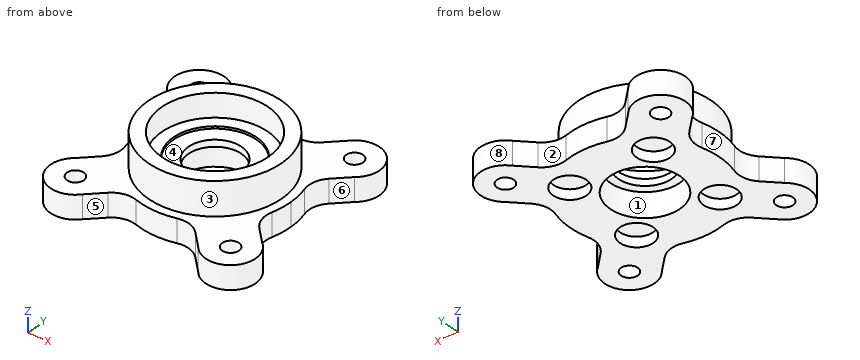
```python
from build123d import *

# Parameters (mm, degrees)
SKETCH1_R                             = 7.5
SKETCH1_R_2                           = 22.5
F_5_IN_SHEET_DEPTH                    = 7
FILLET1_R                             = 7
F_5_0_REAMED_OVER_FOR_SHOULDER_BOLT_D = 5
SKETCH8_R                             = 20
BOSS_EXTRUDE2_DEPTH                   = 10
SKETCH2_R                             = 8
THROUGH_HOLE_DEPTH                    = 47.337664072
SKETCH7_R                             = 10.5
INBOARD_BEARING_CUP_DEPTH             = 7.325
SKETCH11_R                            = 12.5
CUT_EXTRUDE5_DEPTH                    = 7.675
SKETCH12_R                            = 16
CUT_EXTRUDE6_DEPTH                    = 7
SKETCH13_R                            = 5
CUT_EXTRUDE7_DEPTH                    = 3


with BuildPart() as part:
    # Sketch1 → .5 in sheet (new body)
    with BuildSketch(Plane.XY):
        with Locations((22.980970389, 22.980970389)):
            Circle(SKETCH1_R)
        Circle(SKETCH1_R_2)
        with Locations((-22.980970389, 22.980970389)):
            Circle(SKETCH1_R)
        with Locations((-22.980970389, -22.980970389)):
            Circle(SKETCH1_R)
        with Locations((22.980970389, -22.980970389)):
            Circle(SKETCH1_R)
        with BuildLine():
            ThreePointArc((-17.10117153, 27.636930588), (-28.284271247, 28.284271247), (-27.636930588, 17.10117153))
            Line((-27.636930588, 17.10117153), (-17.10117153, 27.636930588))
        make_face()
        with BuildLine():
            Line((-17.10117153, 27.636930588), (-27.636930588, 17.10117153))
            ThreePointArc((-27.636930588, 17.10117153), (-19.715216379, 16.229314981), (-15.480970389, 22.980970389))
            ThreePointArc((-15.480970389, 22.980970389), (-15.897592259, 25.445874906), (-17.10117153, 27.636930588))
        make_face()
        with BuildLine():
            Line((-27.636930588, 17.10117153), (-20.280355849, 9.744596791))
            ThreePointArc((-20.280355849, 9.744596791), (-15.909902577, 15.909902577), (-9.744596791, 20.280355849))
            Line((-9.744596791, 20.280355849), (-17.10117153, 27.636930588))
            ThreePointArc((-17.10117153, 27.636930588), (-15.897592259, 25.445874906), (-15.480970389, 22.980970389))
            ThreePointArc((-15.480970389, 22.980970389), (-19.715216379, 16.229314981), (-27.636930588, 17.10117153))
        make_face()
        with BuildLine():
            Line((-20.280355849, 9.744596791), (-10.535759058, 0))
            Line((-10.535759058, 0), (0, 10.535759058))
            Line((0, 10.535759058), (-9.744596791, 20.280355849))
            ThreePointArc((-9.744596791, 20.280355849), (-15.909902577, 15.909902577), (-20.280355849, 9.744596791))
        make_face()
        with BuildLine():
            Line((-9.744596791, 20.280355849), (0, 10.535759058))
            Line((0, 10.535759058), (9.744596791, 20.280355849))
            ThreePointArc((9.744596791, 20.280355849), (0, 22.5), (-9.744596791, 20.280355849))
        make_face()
        with BuildLine():
            Line((-20.280355849, -9.744596791), (-10.535759058, 0))
            Line((-10.535759058, 0), (-20.280355849, 9.744596791))
            ThreePointArc((-20.280355849, 9.744596791), (-22.5, 0), (-20.280355849, -9.744596791))
        make_face()
        with BuildLine():
            ThreePointArc((-9.744596791, -20.280355849), (0, -22.5), (9.744596791, -20.280355849))
            Line((9.744596791, -20.280355849), (0, -10.535759058))
            Line((0, -10.535759058), (-9.744596791, -20.280355849))
        make_face()
        with BuildLine():
            Line((0, -10.535759058), (9.744596791, -20.280355849))
            ThreePointArc((9.744596791, -20.280355849), (15.909902577, -15.909902577), (20.280355849, -9.744596791))
            Line((20.280355849, -9.744596791), (10.535759058, 0))
            Line((10.535759058, 0), (0, -10.535759058))
        make_face()
        with BuildLine():
            Line((10.535759058, 0), (20.280355849, -9.744596791))
            ThreePointArc((20.280355849, -9.744596791), (21.938072005, -4.997098828), (22.5, 0))
            ThreePointArc((22.5, 0), (21.938072005, 4.997098828), (20.280355849, 9.744596791))
            Line((20.280355849, 9.744596791), (10.535759058, 0))
        make_face()
        with BuildLine():
            Line((0, 10.535759058), (10.535759058, 0))
            Line((10.535759058, 0), (20.280355849, 9.744596791))
            ThreePointArc((20.280355849, 9.744596791), (15.909902577, 15.909902577), (9.744596791, 20.280355849))
            Line((9.744596791, 20.280355849), (0, 10.535759058))
        make_face()
        Polygon((-10.535759058, 0), (0, -10.535759058), (10.535759058, 0), (0, 10.535759058), align=None)
        with BuildLine():
            ThreePointArc((17.10117153, 27.636930588), (17.67766953, 17.67766953), (27.636930588, 17.10117153))
            Line((27.636930588, 17.10117153), (17.10117153, 27.636930588))
        make_face()
        with BuildLine():
            Line((17.10117153, 27.636930588), (27.636930588, 17.10117153))
            ThreePointArc((27.636930588, 17.10117153), (29.732625796, 19.715216379), (30.480970389, 22.980970389))
            ThreePointArc((30.480970389, 22.980970389), (25.445874906, 30.064348518), (17.10117153, 27.636930588))
        make_face()
        with BuildLine():
            ThreePointArc((9.744596791, 20.280355849), (15.909902577, 15.909902577), (20.280355849, 9.744596791))
            Line((20.280355849, 9.744596791), (27.636930588, 17.10117153))
            ThreePointArc((27.636930588, 17.10117153), (17.67766953, 17.67766953), (17.10117153, 27.636930588))
            Line((17.10117153, 27.636930588), (9.744596791, 20.280355849))
        make_face()
        with BuildLine():
            ThreePointArc((27.636930588, -17.10117153), (17.67766953, -17.67766953), (17.10117153, -27.636930588))
            Line((17.10117153, -27.636930588), (27.636930588, -17.10117153))
        make_face()
        with BuildLine():
            Line((27.636930588, -17.10117153), (17.10117153, -27.636930588))
            ThreePointArc((17.10117153, -27.636930588), (25.445874906, -30.064348518), (30.480970389, -22.980970389))
            ThreePointArc((30.480970389, -22.980970389), (29.732625796, -19.715216379), (27.636930588, -17.10117153))
        make_face()
        with BuildLine():
            Line((9.744596791, -20.280355849), (17.10117153, -27.636930588))
            ThreePointArc((17.10117153, -27.636930588), (17.67766953, -17.67766953), (27.636930588, -17.10117153))
            Line((27.636930588, -17.10117153), (20.280355849, -9.744596791))
            ThreePointArc((20.280355849, -9.744596791), (15.909902577, -15.909902577), (9.744596791, -20.280355849))
        make_face()
        with BuildLine():
            ThreePointArc((-27.636930588, -17.10117153), (-28.284271247, -28.284271247), (-17.10117153, -27.636930588))
            Line((-17.10117153, -27.636930588), (-27.636930588, -17.10117153))
        make_face()
        with BuildLine():
            Line((-27.636930588, -17.10117153), (-17.10117153, -27.636930588))
            ThreePointArc((-17.10117153, -27.636930588), (-15.897592259, -25.445874906), (-15.480970389, -22.980970389))
            ThreePointArc((-15.480970389, -22.980970389), (-19.715216379, -16.229314981), (-27.636930588, -17.10117153))
        make_face()
        with BuildLine():
            Line((-17.10117153, -27.636930588), (-9.744596791, -20.280355849))
            ThreePointArc((-9.744596791, -20.280355849), (-15.909902577, -15.909902577), (-20.280355849, -9.744596791))
            Line((-20.280355849, -9.744596791), (-27.636930588, -17.10117153))
            ThreePointArc((-27.636930588, -17.10117153), (-19.715216379, -16.229314981), (-15.480970389, -22.980970389))
            ThreePointArc((-15.480970389, -22.980970389), (-15.897592259, -25.445874906), (-17.10117153, -27.636930588))
        make_face()
    extrude(amount=F_5_IN_SHEET_DEPTH)

    # Fillet1
    fillet1_edges = [part.edges().sort_by_distance(p)[0] for p in [
        (-9.744596791, -20.280355849, 3.5),
        (-20.280355849, -9.744596791, 3.5),
        (-20.280355849, 9.744596791, 3.5),
        (-9.744596791, 20.280355849, 3.5),
        (9.744596791, 20.280355849, 3.5),
        (20.280355849, 9.744596791, 3.5),
        (20.280355849, -9.744596791, 3.5),
        (9.744596791, -20.280355849, 3.5),
    ]]
    fillet(fillet1_edges, radius=FILLET1_R)

    # Ø5.0 Reamed over for shoulder bolt (through all)
    with Locations(Plane(origin=(-11.055401524, 12.777106872, 7), x_dir=(1, 0, 0), z_dir=(0, 0, 1))):
        with Locations((-11.925568864, 10.203863517), (34.036371913, 10.203863517), (34.036371913, -35.758077261), (-11.925568864, -35.758077261)):
            Hole(F_5_0_REAMED_OVER_FOR_SHOULDER_BOLT_D / 2)

    # Sketch8 → Boss-Extrude2 (add)
    with BuildSketch(Plane.XY.offset(7)):
        Circle(SKETCH8_R)
    extrude(amount=BOSS_EXTRUDE2_DEPTH)

    # Sketch2 → Through hole (cut, through all)
    with BuildSketch(Plane.XY):
        Circle(SKETCH2_R)
    extrude(amount=THROUGH_HOLE_DEPTH, mode=Mode.SUBTRACT)

    # Sketch7 → Inboard bearing cup (cut)
    with BuildSketch(Plane(origin=(0, 0, 0), x_dir=(-1, 0, 0), z_dir=(0, 0, -1))):
        Circle(SKETCH7_R)
    extrude(amount=-INBOARD_BEARING_CUP_DEPTH, mode=Mode.SUBTRACT)

    # Sketch11 → Cut-Extrude5 (cut)
    with BuildSketch(Plane.XY.offset(17)):
        Circle(SKETCH11_R)
    extrude(amount=-CUT_EXTRUDE5_DEPTH, mode=Mode.SUBTRACT)

    # Sketch12 → Cut-Extrude6 (cut)
    with BuildSketch(Plane.XY.offset(17)):
        Circle(SKETCH12_R)
    extrude(amount=-CUT_EXTRUDE6_DEPTH, mode=Mode.SUBTRACT)

    # Sketch13 → Cut-Extrude7 (cut)
    with BuildSketch(Plane(origin=(0, 0, 0), x_dir=(-1, 0, 0), z_dir=(0, 0, -1))):
        with Locations((12.374368671, 12.374368671)):
            Circle(SKETCH13_R)
        with Locations((-12.374368671, 12.374368671)):
            Circle(SKETCH13_R)
        with Locations((-12.374368671, -12.374368671)):
            Circle(SKETCH13_R)
        with Locations((12.374368671, -12.374368671)):
            Circle(SKETCH13_R)
    extrude(amount=-CUT_EXTRUDE7_DEPTH, mode=Mode.SUBTRACT)


solid = part.part
```
Verification items for the finished model (mm, model axes). Face numbers are marked on the shaded views. A direction names the side the tool comes from. Round coordinates to 2 decimals unless told otherwise and drop trailing zeros. Write each loop counter-clockwise with the first axis right and the second up, starting at its lowest first coordinate (ties: lowest second). Pieces come first, ordered by that corner, then holes.
1. Scan lines: L1, parallel to Y at x = 24.5, z = 2; L2, parallel to X at y = 0.5, z = 10.25; L3, parallel to Y at x = 24, z = 1. Record each from-to range of solid material in increasing order.
2. Gauge pin test, flat ends, axial feed: P1, Ø3, axis at x = 11, y = 10.5, coming from the -Z side; P2, Ø8, axis at x = -1.5, y = 6, coming from the +Z side (3 decimals); P3, Ø8, axis at x = -22.98, y = 22.98, coming from the +Z side. Record the tip position at first contact, or that the pin passes through.
3. Draft check along Y on the marked faces 1, 2 and 3. Enter one of: +Y half, -Y half, draft (parallel to the pull), parting line (faces both ways), or undercut.
4. Section check B-B on z = 14.5. Enter the section's corners in (x, y).
5. Section check A-A on x = 0. Enter the section's corners in (y, z) (3 decimals), plus the area to 3 significant figures.
6. Section check C-C on y = -11.5. Enter the section's corners in (x, z) (3 decimals).
7. Section check D-D on x = -14.5. Enter the section's corners in (y, z).
8. Access from +Z, -Z, +X, -X, +Y, -Y to the whole of each face (thin tool, end or side, straight path). Record for the marked faces 4, 5, 6, 7 and 8.
Answer:
1. L1: y = -30.33 to -24.97, -21 to -13.96, 13.96 to 21, 24.97 to 30.33
1. L2: x = -19.99 to -15.99, 15.99 to 19.99
1. L3: y = -30.41 to -25.26, -20.7 to -13.46, 13.46 to 20.7, 25.26 to 30.41
2. P1: stops at z = 3
2. P2: stops at z = 9.325
2. P3: stops at z = 7
3. face 1: undercut
3. face 2: +Y half
3. face 3: parting line
4. outline: circle Ø40 at (0, 0); hole circle Ø32 at (0, 0)
5. outline: (-22.5, 0) - (-10.5, 0) - (-10.5, 7.325) - (-8, 7.325) - (-8, 9.325) - (-12.5, 9.325) - (-12.5, 10) - (-16, 10) - (-16, 17) - (-20, 17) - (-20, 7) - (-22.5, 7) - close; (8, 7.325) - (10.5, 7.325) - (10.5, 0) - (22.5, 0) - (22.5, 7) - (20, 7) - (20, 17) - (16, 17) - (16, 10) - (12.5, 10) - (12.5, 9.325) - (8, 9.325) - close
5. area: 288 mm2
6. outline: (-22.36, 0) - (-17.297, 0) - (-17.297, 3) - (-7.451, 3) - (-7.451, 0) - (7.451, 0) - (7.451, 3) - (17.297, 3) - (17.297, 0) - (22.36, 0) - (22.36, 7) - (16.363, 7) - (16.363, 17) - (11.124, 17) - (11.124, 10) - (4.899, 10) - (4.899, 9.325) - (-4.899, 9.325) - (-4.899, 10) - (-11.124, 10) - (-11.124, 17) - (-16.363, 17) - (-16.363, 7) - (-22.36, 7) - close
7. outline: (-25.04, 0) - (-16.9, 0) - (-16.9, 3) - (-7.85, 3) - (-7.85, 0) - (7.85, 0) - (7.85, 3) - (16.9, 3) - (16.9, 0) - (25.04, 0) - (25.04, 7) - (13.77, 7) - (13.77, 17) - (6.76, 17) - (6.76, 10) - (-6.76, 10) - (-6.76, 17) - (-13.77, 17) - (-13.77, 7) - (-25.04, 7) - close
8. face 4: +Z
8. face 5: +Z, -Z, -Y
8. face 6: +Z, -Z, +X
8. face 7: +Z, -Z, -X
8. face 8: +Z, -Z
